from build123d import *


with BuildPart() as part:
    # Sketch1 → Revolve1 (revolve)
    with BuildSketch(Plane.XY):
        Polygon((6.35, 61.087), (5.842, 61.595), (0, 61.595), (0, -61.595), (5.842, -61.595), (6.35, -61.087), (6.35, -58.42), (5.08, -58.42), (5.08, -57.15), (6.35, -57.15), (6.35, -45.72), (5.08, -45.72), (5.08, -44.45), (6.35, -44.45), (6.35, 31.75), (5.08, 31.75), (5.08, 33.02), (6.35, 33.02), (6.35, 57.15), (5.08, 57.15), (5.08, 58.42), (6.35, 58.42), align=None)
    revolve(axis=Axis((0, -61.595, 0), (0, 1, 0)))


solid = part.part
The listing builds one solid part. Answer for the finished solid, in the listing's coordinates (mm). A direction names the side the tool comes from. Give positions to 0.01 mm unless a question says otherwise; leave off trailing zeros. Write each loop counter-clockwise with the first axis right and the second up, starting at its lowest first coordinate (ties: lowest second). Pieces come first, ordered by that corner, then holes. Notation, with made-up numbers: (37, 82) -> (93, 82) arc R27 ccw to (93, 117) -> close; hole circle Ø5 at (19, 76.25). An arc over 180 degrees is marked (long way). Use a Markdown table: item, result.
(1) Determine the mould class of faces 3 (the flat face through (-2, -57.15, -5)), 4 (the cylindrical face through (-1.38, 59.77, 6.2)), 5 (the flat face through (0, -61.595, 0)) for opening direction Y: released by +Y, released by -Y, zero draft, split by the parting line, or undercut.
Return value:
| item | result |
|---|---|
| face 3 | undercut |
| face 4 | zero draft |
| face 5 | released by -Y |
(2) Section A-A, the plane y = 21 is taken. Determine the outline of the cut face in (x, z), then the cut area to 3 significant figures.
Return value:
| item | result |
|---|---|
| outline | circle Ø12.7 at (0, 0) |
| area | 127 mm2 |
(3) For faces 1 (the cylindrical face through (-1.38, -5.82, 6.2)), 2 (the cylindrical face through (-0.661, 32.394, -5.037)), determine the directions among +Z, -Z, +X, -X, +Y, -Y from which every point of the face is accessible in a straight line to the end or side of a thin tool.
Return value:
| item | result |
|---|---|
| face 1 | +Y, -Y |
| face 2 | none |
(4) Flat-ended cylindrical pins translate along their axes: P1, Ø4, axis at x = 3, y = -48.5, coming from the -Z side; P2, Ø1.5, axis at x = -5, y = -25.5, coming from the -Z side. Find the tip coordinate at first contact, or state that the pin passes through.
Return value:
| item | result |
|---|---|
| P1 | z = -6.27 |
| P2 | z = -4.72 |
(5) Find the intervals of material crossed by probe 1 along Y at (x, z) = (5, -1.5) (3 decimals); probe 2 along Z at (x, y) = (2.5, -49); probe 3 along X at (y, z) = (50.5, -0.5), in increasing order. Write a range as from..to.
Return value:
| item | result |
|---|---|
| probe 1 | -61.595..-58.42, -57.15..-45.72, -44.45..31.75, 33.02..57.15, 58.42..61.595 |
| probe 2 | -5.84..5.84 |
| probe 3 | -6.33..6.33 |
